from build123d import *

# Parameters (mm, degrees)
F0_W     = 65
F0_H     = 42
F1_DEPTH = 3
F3_D     = 4.4
F4_D     = 5
F5_R     = 5


with BuildPart() as f1:
    # F0 (on Top) → F1 (new body)
    with BuildSketch(Plane.XY):
        with Locations((32.5, -21)):
            Rectangle(F0_W, F0_H)
    extrude(amount=F1_DEPTH)

    # F3 (through all)
    with Locations(Plane.XY.offset(3)):
        with Locations((10, -10), (10, -32)):
            Hole(F3_D / 2)

    # F4 (through all)
    with Locations(Plane.XY.offset(3)):
        with Locations((44, -21)):
            Hole(F4_D / 2)

    # F5
    f5_edges = [f1.edges().sort_by_distance(p)[0] for p in [
        (0, -42, 1.5),
        (65, -42, 1.5),
        (65, 0, 1.5),
        (0, 0, 1.5),
    ]]
    fillet(f5_edges, radius=F5_R)


solid = f1.part
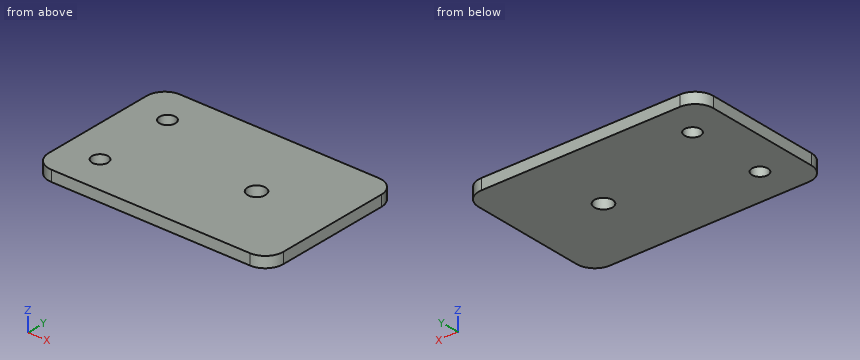
Can you work these out from the model? Positions are in its coordinate system, mm. Give positions to 0.01 mm unless a question says otherwise; leave off trailing zeros. Order: outer loops, then holes, each group sorted by start corner. A loop starts at its lowest first (then second) coordinate and runs counter-clockwise, first axis right, second up. Notation, with made-up numbers: M -12.5,-12.75 L 4.5,-12.75 A26 cw 4.5,1.25 Z; hole C 89.25,-13 d5. An arc over 180 degrees is marked long. Use one line per item in the form item = value. Start each with the question number.
Item 1: If I drill on line 1 along Y through (x, z) = (10, 2); line 2 along Y through (x, z) = (44, 0.7); line 3 along Y through (x, z) = (11.5, 2.45), over which ranges is the centre line in solid material (lowest first)?
Item 2: If we section it at B-B (y = -10): Write out the boundary of the cut face in (x, z), then the cut area to 3 significant figures.
Item 3: If we section it at C-C (z = 2): Write out the boundary of the cut face in (x, y).
Item 4: Will this pin go through, and if not, where does the flat tip stop? pin 1 Ø4 at (x, y) = (10, -32) entering from -Z.
Item 5: If we section it at A-A (x = 10): Write out the boundary of the cut face in (y, z).
Item 6: If we section it at D-D (x = 44): Write out the boundary of the cut face in (y, z).
Outcome:
q1.line_1 = -42 to -34.2, -29.8 to -12.2, -7.8 to 0
q1.line_2 = -42 to -23.5, -18.5 to 0
q1.line_3 = -42 to -33.61, -30.39 to -11.61, -8.39 to 0
q2.outline = M 0,0 L 7.8,0 L 7.8,3 L 0,3 Z; M 12.2,0 L 65,0 L 65,3 L 12.2,3 Z
q2.area = 182 mm2
q3.outline = M 0,-37 A5 ccw 5,-42 L 60,-42 A5 ccw 65,-37 L 65,-5 A5 ccw 60,0 L 5,0 A5 ccw 0,-5 Z; hole C 10,-32 d4.4; hole C 10,-10 d4.4; hole C 44,-21 d5
q4.pin_1 = through
q5.outline = M -42,0 L -34.2,0 L -34.2,3 L -42,3 Z; M -29.8,0 L -12.2,0 L -12.2,3 L -29.8,3 Z; M -7.8,0 L 0,0 L 0,3 L -7.8,3 Z
q6.outline = M -42,0 L -23.5,0 L -23.5,3 L -42,3 Z; M -18.5,0 L 0,0 L 0,3 L -18.5,3 Z
